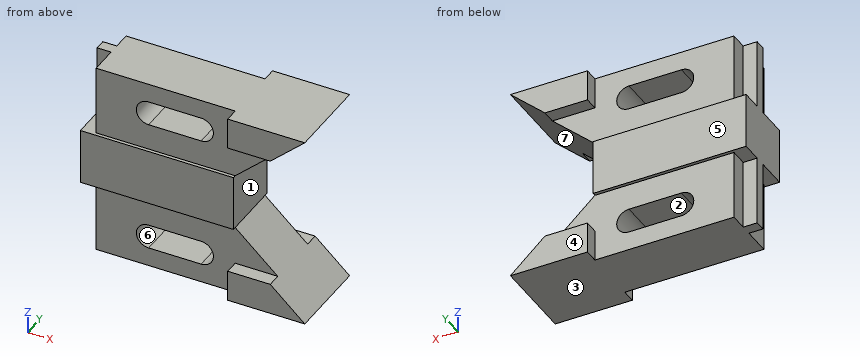
from build123d import *

# Parameters (mm, degrees)
F1_DEPTH = 14.224
F0_W     = 6.35
F0_H     = 17.526
F0_H_2   = 14.224
F2_DEPTH = 4.826
F3_DEPTH = 12.7
F4_DEPTH = 12.7
F5_DEPTH = 19.05


with BuildPart() as f1:
    # F0 (on Front) → F1 (new body, symmetric)
    with BuildSketch(Plane.XZ):
        Polygon((17.272, 12.7), (-45.974, 12.7), (-52.324, 12.7), (-52.324, -12.7), (-45.974, -12.7), (17.272, -12.7), align=None)
    extrude(amount=F1_DEPTH, both=True)

    # F0 (on Front) → F2 (join)
    with BuildSketch(Plane.XZ):
        Polygon((-45.974, 44.45), (-52.324, 44.45), (-52.324, 30.226), (-52.324, 12.7), (-45.974, 12.7), align=None)
        with Locations((-49.149, -21.463)):
            Rectangle(F0_W, F0_H)
        with Locations((-49.149, -37.338)):
            Rectangle(F0_W, F0_H_2)
    extrude(amount=-F2_DEPTH)

    # F0 (on Front) → F3 (join, symmetric)
    with BuildSketch(Plane.XZ):
        Polygon((17.272, 44.45), (-45.974, 44.45), (-45.974, 12.7), (17.272, 12.7), (36.620704, 30.226), (17.272, 30.226), align=None)
        with BuildLine():
            ThreePointArc((-22.098, 24.638), (-27.686, 30.226), (-22.098, 35.814))
            Line((-22.098, 35.814), (1.778, 35.814))
            ThreePointArc((1.778, 35.814), (5.7293126933, 34.1773126933), (7.366, 30.226))
            ThreePointArc((7.366, 30.226), (5.7293126933, 26.2746873067), (1.778, 24.638))
            Line((1.778, 24.638), (-22.098, 24.638))
        make_face(mode=Mode.SUBTRACT)
    extrude(amount=F3_DEPTH, both=True)

    # F0 (on Front) → F4 (join, symmetric)
    with BuildSketch(Plane.XZ):
        Polygon((36.620704, -30.226), (17.272, -12.7), (-45.974, -12.7), (-45.974, -30.226), (-45.974, -44.45), (17.272, -44.45), (17.272, -30.226), align=None)
        with BuildLine():
            ThreePointArc((-22.098, -35.814), (-26.0493126933, -34.1773126933), (-27.686, -30.226))
            ThreePointArc((-27.686, -30.226), (-26.0493126933, -26.2746873067), (-22.098, -24.638))
            Line((-22.098, -24.638), (1.778, -24.638))
            ThreePointArc((1.778, -24.638), (5.7293126933, -26.2746873067), (7.366, -30.226))
            ThreePointArc((7.366, -30.226), (5.7293126933, -34.1773126933), (1.778, -35.814))
            Line((1.778, -35.814), (-22.098, -35.814))
        make_face(mode=Mode.SUBTRACT)
    extrude(amount=F4_DEPTH, both=True)

    # F0 (on Front) → F5 (join, symmetric)
    with BuildSketch(Plane.XZ):
        Polygon((52.324, 44.45), (17.272, 44.45), (17.272, 30.226), (36.620704, 30.226), align=None)
        Polygon((17.272, -44.45), (52.324, -44.45), (36.620704, -30.226), (17.272, -30.226), align=None)
    extrude(amount=F5_DEPTH, both=True)


solid = f1.part
For this review, take the finished solid that the model builds, in its own axes (mm). Face numbers are marked on the shaded views. A direction names the side the tool comes from. Coordinates: 2 decimals unless noted, no trailing zeros. Write each loop counter-clockwise with the first axis right and the second up, starting at its lowest first coordinate (ties: lowest second). Pieces come first, ordered by that corner, then holes. Notation, with made-up numbers: (16.5, -36.5) -> (52.5, -36.5) arc R7 ccw to (52.5, -31.5) -> close; hole circle Ø11 at (72.5, 37.5). An arc over 180 degrees is marked (long way). Write each question's results on one line, items separated by ' | '. Start each with the question number.
1) Consider section B-B (y = -7). Write out the cut boundary in (x, z).
2) Consider section C-C (z = 29). Write out the cut boundary in (x, y).
3) For the marked faces 5, 6 and 7, list the 3-axis set-ups (+Z, -Z, +X, -X, +Y, -Y) from which the entire face can be reached by the end or side of a thin tool; tool diameter is ignored.
4) Consider section D-D (x = -44.5). Write out the cut boundary in (y, z).
5) Wall thickness on L1, parallel to Z at x = 1.5, y = -6; L2, parallel to Z at x = 35.5, y = 17.5; L3, parallel to Z at x = 5, y = -3: over which ranges is each line inside the solid? List them lowest first. Write a range as [from, to].
6) The part is to be moulded in two halves that separate along Z. For the marked faces 1, 2, 3 and 4, say which applies: +Z half, -Z half, draft (parallel to the pull), parting line (faces both ways), or undercut.
7) Insertion check: pin 1 (5 mm diameter, centred on y = -5, z = -19, fed in from +X); pin 2 (4 mm diameter, centred on x = 15.5, z = -10.5, fed in from +Y); pin 3 (10 mm diameter, centred on y = -14.5, z = -11.5, fed in from +X). Each pin has a flat end and moves straight along its axis. Give the tip position at first contact, or say it passes through.
8) Consider section A-A (x = -2). Write out the cut boundary in (y, z).
Geometry says:
1) outline: (-52.32, -12.7) -> (-45.97, -12.7) -> (-45.97, -44.45) -> (52.32, -44.45) -> (17.27, -12.7) -> (17.27, 12.7) -> (52.32, 44.45) -> (-45.97, 44.45) -> (-45.97, 12.7) -> (-52.32, 12.7) -> close; hole (-22.1, -35.81) -> (1.78, -35.81) arc R5.59 ccw to (1.78, -24.64) -> (-22.1, -24.64) arc R5.59 ccw to start; hole (-22.1, 24.64) -> (1.78, 24.64) arc R5.59 ccw to (1.78, 35.81) -> (-22.1, 35.81) arc R5.59 ccw to start
2) outline: (-52.32, 0) -> (-45.97, 0) -> (-45.97, -12.7) -> (-27.55, -12.7) -> (-27.55, 12.7) -> (-45.97, 12.7) -> (-45.97, 4.83) -> (-52.32, 4.83) -> close; (7.23, -12.7) -> (35.27, -12.7) -> (35.27, 12.7) -> (7.23, 12.7) -> close
3) face 5: +Z, -Z, +X, -X, +Y | face 6: +Y, -Y | face 7: +X, +Y, -Y
4) outline: (-14.22, -12.7) -> (-12.7, -12.7) -> (-12.7, -44.45) -> (12.7, -44.45) -> (12.7, -12.7) -> (14.22, -12.7) -> (14.22, 12.7) -> (12.7, 12.7) -> (12.7, 44.45) -> (-12.7, 44.45) -> (-12.7, 12.7) -> (-14.22, 12.7) -> close
5) L1: [-44.45, -35.81], [-24.64, 24.64], [35.81, 44.45] | L2: [-44.45, -30.23], [30.23, 44.45] | L3: [-44.45, -34.79], [-25.66, 25.66], [34.79, 44.45]
6) face 1: undercut | face 2: undercut | face 3: -Z half | face 4: draft
7) pin 1: x = 26.99 | pin 2: y = 14.22 | pin 3: x = 21.1
8) outline: (-14.22, -12.7) -> (-12.7, -12.7) -> (-12.7, -24.64) -> (12.7, -24.64) -> (12.7, -12.7) -> (14.22, -12.7) -> (14.22, 12.7) -> (12.7, 12.7) -> (12.7, 24.64) -> (-12.7, 24.64) -> (-12.7, 12.7) -> (-14.22, 12.7) -> close; (-12.7, -44.45) -> (12.7, -44.45) -> (12.7, -35.81) -> (-12.7, -35.81) -> close; (-12.7, 35.81) -> (12.7, 35.81) -> (12.7, 44.45) -> (-12.7, 44.45) -> close
